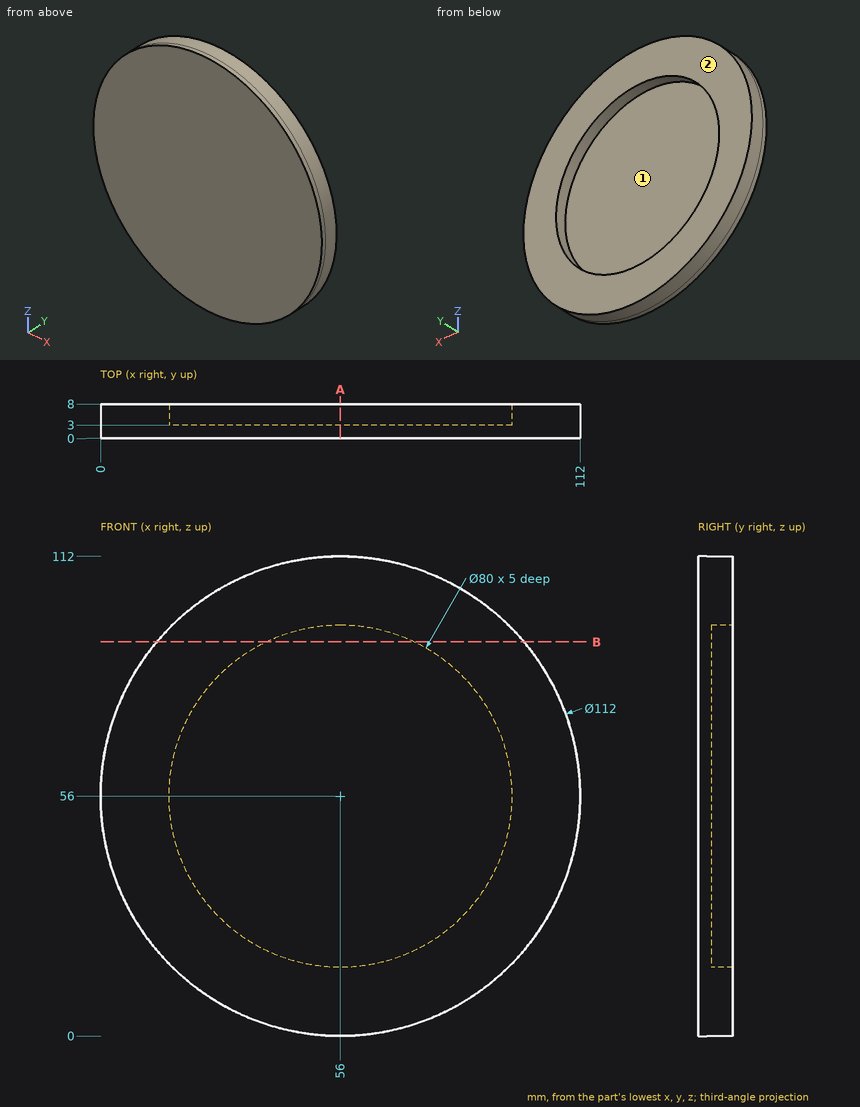
Source: three-view drawing plus pictorial views. Frame: mm from the lowest corner of the part. Round coordinates to 2 decimals unless told otherwise and drop trailing zeros. Write each loop counter-clockwise with the first axis right and the second up, starting at its lowest first coordinate (ties: lowest second). Pieces come first, ordered by that corner, then holes. Notation, with made-up numbers: M -17,-26 L 1,-26 A28 cw 1,0 Z; hole C 64.25,2 d11. An arc over 180 degrees is marked long. Use CSV: the item, a comma, the result in double quotes. Start each with the question number.
Q1. Cut plane A-A on x = 56. Output: boundary loops of the cut face in (y, z).
Q2. First-contact query: P1, Ø5, axis at x = 46.5, z = 58, coming from the +Y side; P2, Ø8, axis at x = 86, z = 83, coming from the -Y side; P3, Ø1, axis at y = 3, z = 14, coming from the -X side; P4, Ø2, axis at y = 5.5, z = 65.5, coming from the +X side. Flat tips, straight axial feed; report the tip coordinate or a pass-through.
Q3. Pull-direction query (Z, two-part tool) for the marked faces 1 and 2; classes: +Z half, -Z half, draft (parallel to the pull), parting line (faces both ways), or undercut.
Q4. Line query: line 1 (X direction, y = 5.65, z = 56); line 2 (Y direction, x = 48, z = 37); line 3 (X direction, y = 4.25, z = 34). Output: solid intervals per line, ascending. Write a range as from..to.
Q5. Cut plane B-B on z = 92. Output: boundary loops of the cut face in (x, y).
Results found:
1,outline,"M 0,0 L 8,0 L 8,16 L 3,16 L 3,96 L 8,96 L 8,112 L 0,112 Z"
2,P1,"y = 3"
2,P2,"y = 0"
2,P3,"x = 18.4"
2,P4,"x = 111.35"
3,face 1,"undercut"
3,face 2,"draft"
4,line 1,"0..16, 96..112"
4,line 2,"0..3"
4,line 3,"4.5..22.59, 89.41..107.5"
5,outline,"M 13.1,0 L 98.9,0 L 98.9,8 L 73.44,8 L 73.44,3 L 38.56,3 L 38.56,8 L 13.1,8 Z"
